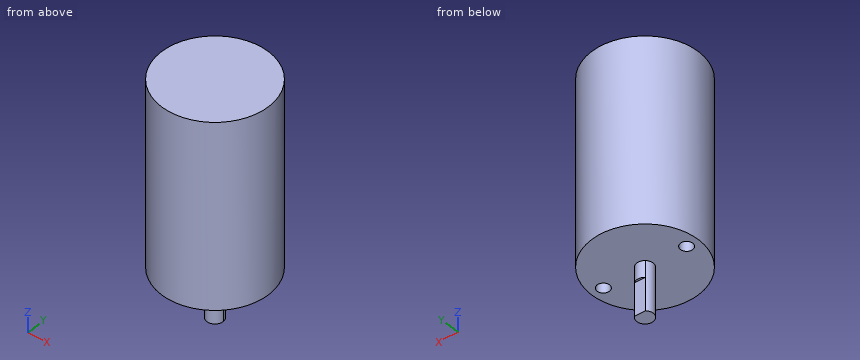
from build123d import *

# Parameters (mm, degrees)
SKETCH1_R                 = 13
MOTOR_BODY_DEPTH          = 45
BOSS_EXTRUDE2_DEPTH       = 12
BOSS_EXTRUDE3_DEPTH       = 4
F_3_0MM_DOWEL_HOLE2_D     = 3
F_3_0MM_DOWEL_HOLE2_DEPTH = 5
F_3_0MM_DOWEL_HOLE2_TIP   = 0.901290929


with BuildPart() as part:
    # Sketch1 → Motor Body (new body)
    with BuildSketch(Plane.XY):
        with Locations(Location((0, 0, 0), (0, 0, 180))):
            Circle(SKETCH1_R)
    extrude(amount=MOTOR_BODY_DEPTH)

    # Sketch2 → Boss-Extrude2 (add)
    with BuildSketch(Plane.XY):
        with BuildLine():
            ThreePointArc((2, 0), (1.822875656, 0.822875656), (1.322875656, 1.5))
            Line((1.322875656, 1.5), (-1.322875656, 1.5))
            ThreePointArc((-1.322875656, 1.5), (-0.822875656, -1.822875656), (2, 0))
        make_face()
    extrude(amount=-BOSS_EXTRUDE2_DEPTH)

    # Sketch2<3> → Boss-Extrude3 (add)
    with BuildSketch(Plane.XY):
        with BuildLine():
            ThreePointArc((2, 0), (1.822875656, 0.822875656), (1.322875656, 1.5))
            Line((1.322875656, 1.5), (-1.322875656, 1.5))
            ThreePointArc((-1.322875656, 1.5), (-0.822875656, -1.822875656), (2, 0))
        make_face()
        with BuildLine():
            Line((-1.322875656, 1.5), (1.322875656, 1.5))
            ThreePointArc((1.322875656, 1.5), (0, 2), (-1.322875656, 1.5))
        make_face()
    extrude(amount=-BOSS_EXTRUDE3_DEPTH)

    # Ø3.0mm Dowel Hole2
    with Locations(Plane(origin=(0, 0, 0), x_dir=(-1, 0, 0), z_dir=(0, 0, -1))):
        with Locations((-10, 0), (10, 0)):
            Hole(F_3_0MM_DOWEL_HOLE2_D / 2, depth=F_3_0MM_DOWEL_HOLE2_DEPTH)
            with Locations((0, 0, -(F_3_0MM_DOWEL_HOLE2_DEPTH + F_3_0MM_DOWEL_HOLE2_TIP / 2))):  # 118° drill point
                Cone(0, F_3_0MM_DOWEL_HOLE2_D / 2, F_3_0MM_DOWEL_HOLE2_TIP, mode=Mode.SUBTRACT)


solid = part.part
Input: part model. Units: mm. Frame: model coordinates. Give positions to 0.01 mm unless a question says otherwise; leave off trailing zeros. Loops run counter-clockwise (first coordinate to the right, second up) from the corner with the lowest first, then second, coordinate; pieces in that order, holes last. Notation, with made-up numbers: (11, 61) - (28, 61) arc R30 ccw to (28, 99) - close; hole circle Ø2 at (61.5, -39). An arc over 180 degrees is marked (long way). Use CSV: the item, a comma, the result in double quotes. Start each with the question number.
Item 1: Line query: line 1 (Z direction, x = -11, y = 4.5); line 2 (Y direction, x = 10, z = 1.55); line 3 (Y direction, x = 0, z = 17.5). Output: solid intervals per line, ascending.
Item 2: Section C-C on y = -7. Return loops of the section in (x, z), then the cut area to 3 significant figures.
Item 3: Section D-D on y = 11. Return loops of the section in (x, z), then the cut area to 3 significant figures.
Item 4: Section B-B on z = 2. Return loops of the section in (x, y).
Item 5: Contact query for flat-ended pins moving along their axis: P1, Ø1, axis at x = -6.5, z = 37.5, coming from the +Y side; P2, Ø3, axis at y = 7, z = -3, coming from the +X side; P3, Ø1.8, axis at x = -10, y = 0, coming from the -Z side; P4, Ø2, axis at x = -3, z = 6, coming from the +Y side. Output: stop coordinate, or through.
Item 6: Section A-A on x = 0. Return loops of the section in (y, z).
Ans:
1,line 1,"z = 0 to 45"
1,line 2,"y = -8.31 to -1.5, 1.5 to 8.31"
1,line 3,"y = -13 to 13"
2,outline,"(-10.95, 0) - (10.95, 0) - (10.95, 45) - (-10.95, 45) - close"
2,area,"986 mm2"
3,outline,"(-6.93, 0) - (6.93, 0) - (6.93, 45) - (-6.93, 45) - close"
3,area,"624 mm2"
4,outline,"circle Ø26 at (0, 0); hole circle Ø3 at (-10, 0); hole circle Ø3 at (10, 0)"
5,P1,"stops at y = 11.53"
5,P2,"passes through"
5,P3,"stops at z = 5.36"
5,P4,"stops at y = 12.85"
6,outline,"(-13, 0) - (-2, 0) - (-2, -12) - (1.5, -12) - (1.5, -4) - (2, -4) - (2, 0) - (13, 0) - (13, 45) - (-13, 45) - close"
